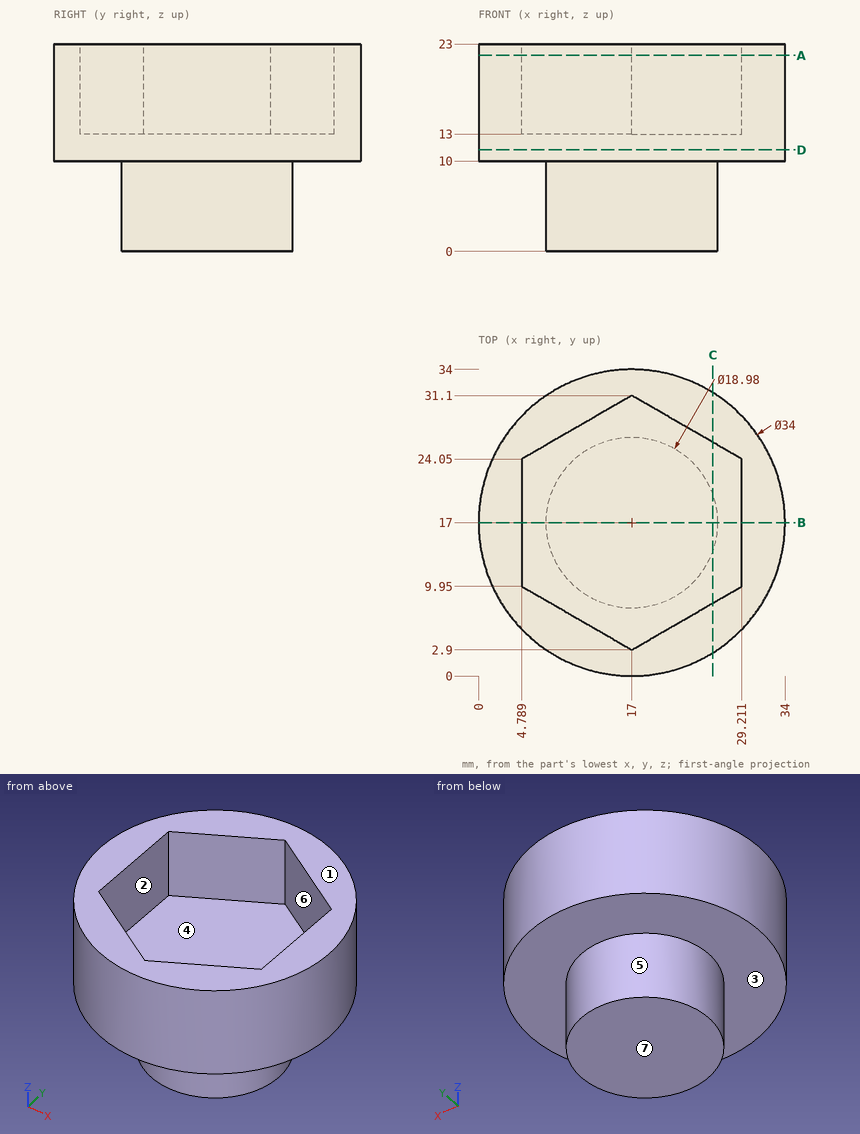
Input: dimensioned drawing with shaded views. Units: mm. Origin: part minimum x, y, z. A direction names the side the tool comes from. Round coordinates to 2 decimals unless told otherwise and drop trailing zeros. Loops run counter-clockwise (first coordinate to the right, second up) from the corner with the lowest first, then second, coordinate; pieces in that order, holes last. Notation, with made-up numbers: (58, 40) -> (91, 40) arc R23 ccw to (91, 71) -> close; hole circle Ø1 at (-23, 29). An arc over 180 degrees is marked (long way). Answer as a JSON object with one key per item and string values. Group by question number.
Q1. Section query C-C (x = 26). Output: boundary loops of the cut face in (y, z), plus the area to 3 significant figures.
Q2. Section query A-A (z = 21.75). Output: boundary loops of the cut face in (x, y), plus the area to 3 significant figures.
Q3. Section query D-D (z = 11.25). Output: boundary loops of the cut face in (x, y).
Q4. Section query B-B (y = 17). Output: boundary loops of the cut face in (x, z).
Q5. Ray query, line 1 (Z direction, x = 18.5, y = 11); line 2 (Z direction, x = 9.5, y = 10.5); line 3 (Y direction, x = 20.5, z = 15.75). Return the intervals inside material, ascending. Write a range as from..to.
Q6. Mould query, pull axis Y, two halves, no side actions, for the marked faces 4, 5, 6 and 7. Classes: pulls with the +Y half, pulls with the -Y half, needs draft (parallel to the pull), parting line crosses it, or undercut.
Q7. Contact query for flat-ended pins moving along their axis: P1, Ø2, axis at y = 7, z = 12, coming from the +X side; P2, Ø1.5, axis at x = 14.5, y = 28, coming from the -Z side; P3, Ø8, axis at x = 27.5, z = 19.5, coming from the -Y side. Output: stop coordinate, or through.
Q8. Access query for the marked faces 1, 2 and 3. Directions: +Z, -Z, +X, -X, +Y, -Y. A direction counts if a zero-diameter tool reaches every point of the face in a straight line with its end or side. Return the directions, or none.
Completed:
{
 "1": {"outline": "(2.58, 10) -> (13.99, 10) -> (13.99, 0) -> (20.01, 0) -> (20.01, 10) -> (31.42, 10) -> (31.42, 23) -> (25.9, 23) -> (25.9, 13) -> (8.1, 13) -> (8.1, 23) -> (2.58, 23) -> close", "area": "257 mm²"},
 "2": {"outline": "circle Ø34 at (17, 17); hole (4.79, 9.95) -> (17, 2.9) -> (29.21, 9.95) -> (29.21, 24.05) -> (17, 31.1) -> (4.79, 24.05) -> close", "area": "391 mm²"},
 "3": {"outline": "circle Ø34 at (17, 17)"},
 "4": {"outline": "(0, 10) -> (7.51, 10) -> (7.51, 0) -> (26.49, 0) -> (26.49, 10) -> (34, 10) -> (34, 23) -> (29.21, 23) -> (29.21, 13) -> (4.79, 13) -> (4.79, 23) -> (0, 23) -> close"},
 "5": {"line 1": "0..13", "line 2": "10..13", "line 3": "0.36..4.92, 29.08..33.64"},
 "6": {"face 4": "undercut", "face 5": "parting line crosses it", "face 6": "undercut", "face 7": "needs draft"},
 "7": {"P1": "x = 31.42", "P2": "z = 10", "P3": "y = 1.29"},
 "8": {"face 1": "+Z, +X, -X, +Y, -Y", "face 2": "+Z", "face 3": "-Z"}
}
